Can you work these out from the drawing? Everything is in mm from the part's minimum corner. A direction names the side the tool comes from. Coordinates: 2 decimals unless noted, no trailing zeros. Write each loop counter-clockwise with the first axis right and the second up, starting at its lowest first coordinate (ties: lowest second). Pieces come first, ordered by that corner, then holes. Notation, with made-up numbers: M -34,-37.5 L -15,-37.5 A17 cw -15,-31.5 Z; hole C -21,40.25 d10. An arc over 180 degrees is marked long. Write each question's results on one line, items separated by ' | '. Start each with the question number.
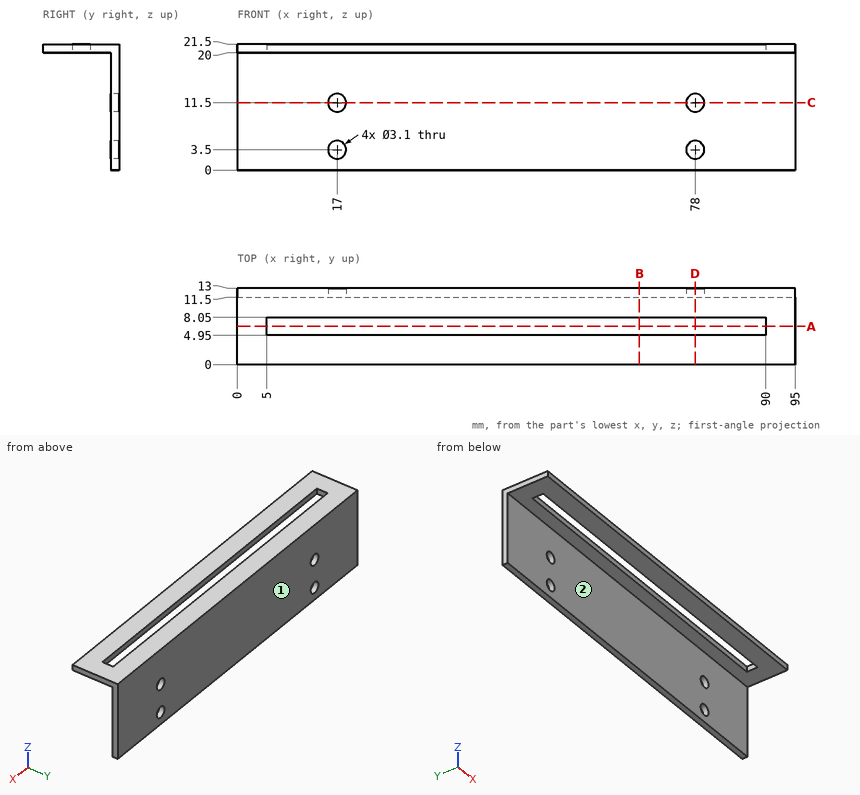
1) I want a section at D-D, the plane x = 78. Write out the boundary of the cut face in (y, z), then the cut area to 4 significant figures.
2) For the marked faces 1 and 2, which set-ups out of +Z, -Z, +X, -X, +Y, -Y let a thin tool reach every point of the face, with its end or its side?
3) For pin 1 Ø4 at (x, y) = (69.5, 1.5) entering from -Z; pin 2 Ø3 at (y, z) = (8, 17) entering from +X, each with a flat end and sliding along its axis, tell me the tip position at first contact or that it passes through.
4) Please list where these lines run through material, in increasing order: line 1 (X direction, y = 12.25, z = 11.5); line 2 (Z direction, x = 17, y = 12); line 3 (Z direction, x = 56, y = 10.25). Write a range as [from, to].
5) I want a section at A-A, the plane y = 6.5. Write out the boundary of the cut face in (x, z).
6) I want a section at B-B, the plane x = 68.5. Write out the boundary of the cut face in (y, z).
7) I want a section at C-C, the plane z = 11.5. Write out the boundary of the cut face in (x, y).
Output:
1) outline: M 0,20 L 4.95,20 L 4.95,21.5 L 0,21.5 Z; M 8.05,20 L 11.5,20 L 11.5,13.05 L 13,13.05 L 13,21.5 L 8.05,21.5 Z; M 11.5,0 L 13,0 L 13,1.95 L 11.5,1.95 Z; M 11.5,5.05 L 13,5.05 L 13,9.95 L 11.5,9.95 Z | area: 35.55 mm2
2) face 1: +Z, -Z, +X, -X, +Y | face 2: -Z, +X, -X, -Y
3) pin 1: stops at z = 20 | pin 2: passes through
4) line 1: x = [0, 15.45], [18.55, 76.45], [79.55, 95] | line 2: z = [0, 1.95], [5.05, 9.95], [13.05, 21.5] | line 3: z = [20, 21.5]
5) outline: M 0,20 L 5,20 L 5,21.5 L 0,21.5 Z; M 90,20 L 95,20 L 95,21.5 L 90,21.5 Z
6) outline: M 0,20 L 4.95,20 L 4.95,21.5 L 0,21.5 Z; M 8.05,20 L 11.5,20 L 11.5,0 L 13,0 L 13,21.5 L 8.05,21.5 Z
7) outline: M 0,11.5 L 15.45,11.5 L 15.45,13 L 0,13 Z; M 18.55,11.5 L 76.45,11.5 L 76.45,13 L 18.55,13 Z; M 79.55,11.5 L 95,11.5 L 95,13 L 79.55,13 Z
